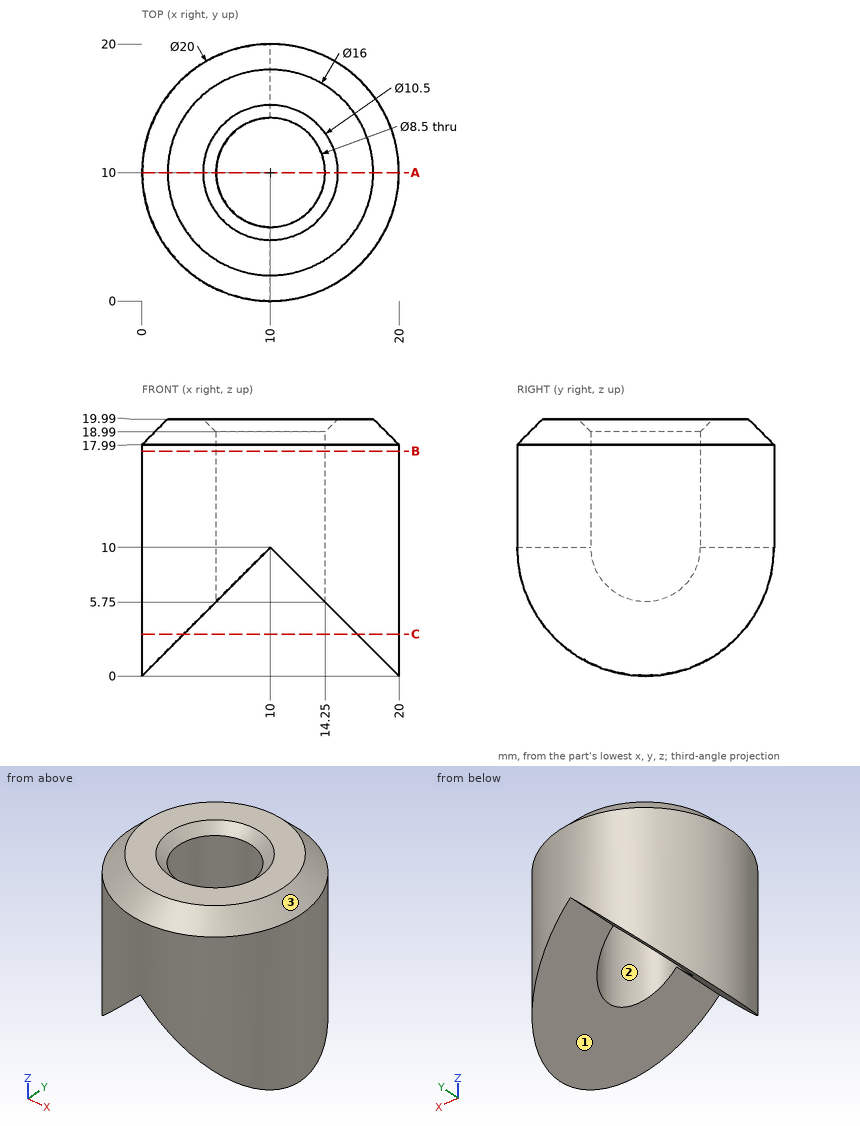
Geometry check sheet. Reference: drawing and pictorial views, mm from the part's lowest x, y, z. Give positions to 0.01 mm unless a question says otherwise; leave off trailing zeros. Order: outer loops, then holes, each group sorted by start corner. A loop starts at its lowest first (then second) coordinate and runs counter-clockwise, first axis right, second up. Notation, with made-up numbers: (-15.5, 8.25) - (18.5, 8.25) arc R34 ccw to (18.5, 45.25) - close; hole circle Ø4 at (76.25, 78). An arc over 180 degrees is marked (long way). Use one line per item in the form item = value.
1) Sectioned sample at A-A (y = 10). Record the boundary of the cut face in (x, z).
Working result:
outline = (0, 0) - (5.75, 5.75) - (5.75, 18.99) - (4.75, 19.99) - (2, 19.99) - (0, 17.99) - close; (14.25, 5.75) - (20, 0) - (20, 17.99) - (18, 19.99) - (15.25, 19.99) - (14.25, 18.99) - close
2) Depth check by flat-ended pin: pin 1 Ø1.5 at (x, y) = (11.5, 10.5) entering from +Z; pin 2 Ø8 at (x, y) = (7, 8) entering from -Z; pin 3 Ø3 at (y, z) = (13.5, 3) entering from +X; pin 4 Ø4 at (y, z) = (14.5, 3.5) entering from -X. Enter the tip coordinate at first touch or a pass-through.
Working result:
pin_1 = through
pin_2 = 3
pin_3 = 19.8
pin_4 = 0.32
3) Sectioned sample at B-B (z = 17.5). Record the boundary of the cut face in (x, y), and give its area (3 significant figures).
Working result:
outline = circle Ø20 at (10, 10); hole circle Ø8.5 at (10, 10)
area = 257 mm^2
4) Sectioned sample at C-C (z = 3.25). Record the boundary of the cut face in (x, y).
Working result:
outline = (3.25, 2.62) - (3.25, 17.38) arc R10 ccw to start; (16.75, 2.62) arc R10 ccw to (16.75, 17.38) - close
5) Material ranges on probe 1 along X at (y, z) = (10, 9.5); probe 2 along X at (y, z) = (13, 13.25), recorded low to high. Write a range as from..to.
Working result:
probe_1 = 0..5.75, 14.25..20
probe_2 = 0.46..6.99, 13.01..19.54
6) Draft check along Y on the marked faces 1, 2 and 3. Enter one of: released by +Y, released by -Y, zero draft, split by the parting line, or undercut.
Working result:
face_1 = zero draft
face_2 = undercut
face_3 = split by the parting line
